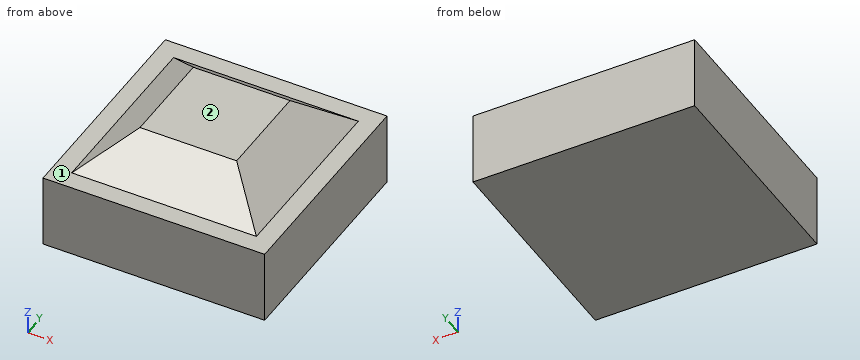
```python
from build123d import *

# Parameters (mm, degrees)
F0_W     = 76.2
F0_H     = 76.2
F1_DEPTH = 25.4
F2_W     = 63.5
F2_H     = 63.5
F3_DEPTH = 12.7
F4_SIZE2 = 15.135261
F4_SIZE  = 12.69999


# Not quite as in the source:
# - a fillet or chamfer is up to 0.001 mm smaller than in the source, because OpenCascade refuses the exact size


with BuildPart() as f1:
    # F0 (on Top) → F1 (new body)
    with BuildSketch(Plane.XY):
        Rectangle(F0_W, F0_H)
    extrude(amount=F1_DEPTH)

    # F2 (on face) → F3 (join)
    with BuildSketch(Plane.XY.offset(25.4)):
        Rectangle(F2_W, F2_H)
    extrude(amount=F3_DEPTH)

    # F4 (size 12.7 and 15.1352706259 in the source; OpenCascade refuses exactly that, so slightly less here)
    f4_edges = [f1.edges().sort_by_distance(p)[0] for p in [
        (0, -31.75, 38.1),
        (-31.75, 0, 38.1),
        (0, 31.75, 38.1),
        (31.75, 0, 38.1),
    ]]
    chamfer(f4_edges, length=F4_SIZE, length2=F4_SIZE2)


solid = f1.part
```
Geometry check sheet. Reference: the model listing, model coordinates, mm. Face numbers are marked on the shaded views. A direction names the side the tool comes from. Coordinates: 2 decimals unless noted, no trailing zeros. Loops run counter-clockwise (first coordinate to the right, second up) from the corner with the lowest first, then second, coordinate; pieces in that order, holes last.
Item 1: Sectioned sample at D-D, the plane x = 33. Record the boundary of the cut face in (y, z), then the cut area to 3 significant figures.
Item 2: Access from +Z, -Z, +X, -X, +Y, -Y to the whole of each face (thin tool, end or side, straight path). Record for the marked faces 1 and 2.
Item 3: Sectioned sample at C-C, the plane z = 30. Record the boundary of the cut face in (x, y), then the cut area to 3 significant figures.
Item 4: Go/stop test with flat-tipped pins: pin 1 Ø1.5 at (x, y) = (29.5, -7) entering from +Z; pin 2 Ø1.5 at (x, z) = (-15.5, 34) entering from -Y; pin 3 Ø5 at (x, y) = (-29, -7.5) entering from +Z. Record where each tip stops, or that it passes through.
Item 5: Thickness scan on line 1 (Z direction, x = 35, y = -31); line 2 (X direction, y = -15, z = 26.5); line 3 (Z direction, x = -18, y = 3). Record the ranges inside material, lowest first.
Check result:
1. outline: (-38.1, 0) - (38.1, 0) - (38.1, 25.4) - (-38.1, 25.4) - close
1. area: 1,940 mm2
2. face 1: +Z
2. face 2: +Z, +X, -X, +Y, -Y
3. outline: (-26.27, -26.27) - (26.27, -26.27) - (26.27, 26.27) - (-26.27, 26.27) - close
3. area: 2,760 mm2
4. pin 1: stops at z = 27.92
4. pin 2: stops at y = -22.39
4. pin 3: stops at z = 29.81
5. line 1: z = 0 to 25.4
5. line 2: x = -30.44 to 30.44
5. line 3: z = 0 to 36.94
